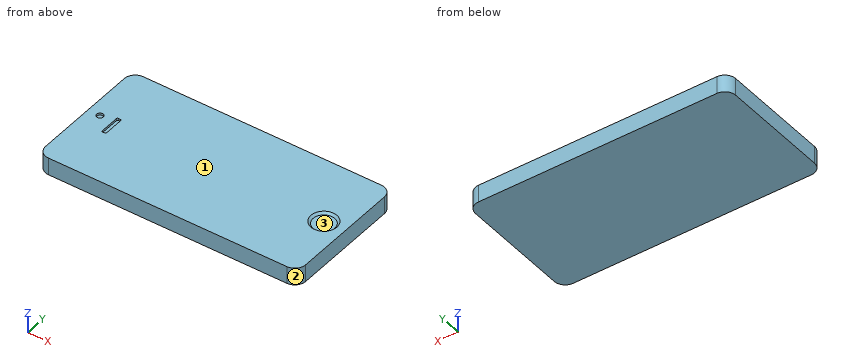
from build123d import *

# Parameters (mm, degrees)
F0_W      = 120
F0_H      = 60
F1_DEPTH  = 8
F2_R      = 5
F3_R      = 5
F4_R      = 5
F5_R      = 5
F6_W      = 2
F6_H      = 10
F7_DEPTH  = 1
F8_R      = 0.5
F9_R      = 0.5
F10_R     = 1.5
F11_DEPTH = 1
F14_R     = 6
F15_DEPTH = 1
F16_SIZE  = 0.99999


# Not quite as in the source:
# - a fillet or chamfer is up to 0.001 mm smaller than in the source, because OpenCascade refuses the exact size


with BuildPart() as f1:
    # F0 (on Top) → F1 (new body)
    with BuildSketch(Plane.XY):
        with Locations((60, 30)):
            Rectangle(F0_W, F0_H)
    extrude(amount=F1_DEPTH)

    # F2
    f2_edges = [f1.edges().sort_by_distance(p)[0] for p in [
        (0, 60, 4),
    ]]
    fillet(f2_edges, radius=F2_R)

    # F3
    f3_edges = [f1.edges().sort_by_distance(p)[0] for p in [
        (0, 0, 4),
    ]]
    fillet(f3_edges, radius=F3_R)

    # F4
    f4_edges = [f1.edges().sort_by_distance(p)[0] for p in [
        (120, 0, 4),
    ]]
    fillet(f4_edges, radius=F4_R)

    # F5
    f5_edges = [f1.edges().sort_by_distance(p)[0] for p in [
        (120, 60, 4),
    ]]
    fillet(f5_edges, radius=F5_R)

    # F6 (on face) → F7 (cut)
    with BuildSketch(Plane.XY.offset(8)):
        with Locations((12.6586212461, 29.4524356723)):
            Rectangle(F6_W, F6_H)
    extrude(amount=-F7_DEPTH, mode=Mode.SUBTRACT)

    # F8
    f8_edges = [f1.edges().sort_by_distance(p)[0] for p in [
        (11.658621, 24.452436, 7.5),
        (13.658621, 24.452436, 7.5),
    ]]
    fillet(f8_edges, radius=F8_R)

    # F9
    f9_edges = [f1.edges().sort_by_distance(p)[0] for p in [
        (13.658621, 34.452436, 7.5),
        (11.658621, 34.452436, 7.5),
    ]]
    fillet(f9_edges, radius=F9_R)

    # F10 (on face) → F11 (cut)
    with BuildSketch(Plane.XY.offset(8)):
        with Locations((5.6273336522, 31.8058170378)):
            Circle(F10_R)
    extrude(amount=-F11_DEPTH, mode=Mode.SUBTRACT)

    # F14 (on face) → F15 (cut)
    with BuildSketch(Plane.XY.offset(8)):
        with Locations((110.2445796132, 30)):
            Circle(F14_R)
    extrude(amount=-F15_DEPTH, mode=Mode.SUBTRACT)

    # F16 (size 1 in the source; OpenCascade refuses exactly that, so slightly less here)
    f16_edges = [f1.edges().sort_by_distance(p)[0] for p in [
        (104.24458, 30, 7),
    ]]
    chamfer(f16_edges, length=F16_SIZE)


solid = f1.part
Here's how the part is built. I have some questions about the finished solid (model axes, mm). Face numbers are marked on the shaded views. Coordinates: 2 decimals unless noted, no trailing zeros. Use CSV: the item, a comma, the result in double quotes. Start each with the question number.
1. Please list where these lines run through material, in increasing order: line 1 (X direction, y = 28.5, z = 7.5); line 2 (X direction, y = 56.5, z = 2.75). Write a range as from..to.
2. If we mould it in two halves opening along Y, with no side actions, what happens to the marked faces 1, 2 and 3? For each: +Y half, -Y half, draft (parallel to the pull), parting line (faces both ways), or undercut.
3. I'm going to push a flat-ended pin straight in: pin 1 (0.9 mm diameter, centred on x = 5, y = 31.5, fed in from +Z). Where does the tip first touch, or does it pass through?
Output:
1,line 1,"x = 0..11.66, 13.66..104.95, 115.54..120"
1,line 2,"x = 0.23..119.77"
2,face 1,"draft"
2,face 2,"-Y half"
2,face 3,"undercut"
3,pin 1,"stops at z = 7"
